Read the model definition and answer for the solid it produces. Units are mm, in the model's axes. A direction names the side the tool comes from. Round coordinates to 2 decimals unless told otherwise and drop trailing zeros. Order: outer loops, then holes, each group sorted by start corner. A loop starts at its lowest first (then second) coordinate and runs counter-clockwise, first axis right, second up. Notation, with made-up numbers: (12.5, 30) -> (61.5, 30) arc R19 cw to (61.5, 44) -> close; hole circle Ø9 at (7, 74). An arc over 180 degrees is marked (long way). Answer as a JSON object with one key per item and string values. Group by question number.
Item 1: Section C-C, the plane z = -15.75 is taken. Write down the section's boundary in (x, y), plus the area to 3 significant figures.
Item 2: For faces 1 (the flat face through (12.7, 72, -17)), 2 (the flat face through (-0.7, 5.1, -23)), 3 (the cylindrical face through (1.653, 121.812, -20.372)), determine the directions among +Z, -Z, +X, -X, +Y, -Y from which every point of the face is accessible in a straight line to the end or side of a thin tool.
Item 3: Section B-B, the plane z = -22.5 is taken. Write down the section's boundary in (x, y).
Item 4: The mould has two halves that part along Y. Classify faces 4 (the cylindrical face through (1.38, 103.02, -18.96)), 5 (the cylindrical face through (20.3, 14.9, -16.5)), 6 (the flat face through (0, 61, -12.7)): pulls with the +Y half, pulls with the -Y half, needs draft (parallel to the pull), parting line crosses it, or undercut.
Item 5: Consider probe 1 along X at (y, z) = (78, -17.5); probe 2 along Z at (x, y) = (5, 35); probe 3 along Y at (x, z) = (0, -17). Determine where each line is inside the solid, lowest interval first. Write a range as from..to.
Item 6: Section D-D, the plane y = 100.5 is taken. Write down the section's boundary in (x, z).
Item 7: Given P1, Ø1.5, axis at x = -39, z = -18, coming from the +Y side; P2, Ø12, axis at x = 12, y = 27, coming from the -Z side; P3, Ø14.5, axis at x = 0, y = 109.22, coming from the +Z side; P4, Ø4, axis at y = 72, z = -16, coming from the +X side, each flat-ended and moving along its own axis, determine where each tip first touches the part or whether it passes through.
from build123d import *

# Parameters (mm, degrees)
SKETCH1_R           = 6.35
BOSS_EXTRUDE1_DEPTH = 7.62
BOSS_EXTRUDE2_START = -5.08
SKETCH4_R           = 12.7
SKETCH4_R_2         = 6.35
BOSS_EXTRUDE2_DEPTH = 7.62
BOSS_EXTRUDE3_START = -5.08
SKETCH4_3_R         = 12.7
SKETCH4_3_R_2       = 6.35
BOSS_EXTRUDE3_DEPTH = 5.08
FILLET1_R           = 25.4
CHAMFER1_SIZE       = 4.92
CUT_EXTRUDE1_DEPTH  = 161.724006919


with BuildPart() as part:
    # Sketch1 → Boss-Extrude1 (new body)
    with BuildSketch(Plane(origin=(0, 0, 0), x_dir=(1, 0, 0), z_dir=(0, 1, 0))):
        with BuildLine():
            Line((-50.8, 25.4), (50.8, 25.4))
            Line((50.8, 25.4), (50.8, 0))
            ThreePointArc((50.8, 0), (43.360512242, -17.960512242), (25.4, -25.4))
            Line((25.4, -25.4), (-25.4, -25.4))
            ThreePointArc((-25.4, -25.4), (-43.360512242, -17.960512242), (-50.8, 0))
            Line((-50.8, 0), (-50.8, 25.4))
        make_face()
        with Locations(Location((-25.4, 0, 0), (0, 0, 90))):
            Circle(SKETCH1_R, mode=Mode.SUBTRACT)
        with Locations(Location((25.4, 0, 0), (0, 0, 90))):
            Circle(SKETCH1_R, mode=Mode.SUBTRACT)
    extrude(amount=BOSS_EXTRUDE1_DEPTH)

    # Sketch4 → Boss-Extrude2 (add)
    with BuildSketch(Plane(origin=(0, 0, -25.4), x_dir=(-1, 0, 0), z_dir=(0, 0, -1)).offset(BOSS_EXTRUDE2_START)):
        with BuildLine():
            Line((12.7, 7.62), (12.7, 109.22))
            ThreePointArc((12.7, 109.22), (0, 96.52), (-12.7, 109.22))
            Line((-12.7, 109.22), (-12.7, 7.62))
            Line((-12.7, 7.62), (12.7, 7.62))
        make_face()
        with Locations((0, 109.22)):
            Circle(SKETCH4_R)
        with Locations((0, 109.22)):
            Circle(SKETCH4_R_2, mode=Mode.SUBTRACT)
    extrude(amount=-BOSS_EXTRUDE2_DEPTH)

    # Sketch4_3 → Boss-Extrude3 (add)
    with BuildSketch(Plane(origin=(0, 0, -25.4), x_dir=(-1, 0, 0), z_dir=(0, 0, -1)).offset(BOSS_EXTRUDE3_START)):
        with Locations((0, 109.22)):
            Circle(SKETCH4_3_R)
        with Locations((0, 109.22)):
            Circle(SKETCH4_3_R_2, mode=Mode.SUBTRACT)
    extrude(amount=BOSS_EXTRUDE3_DEPTH)

    # Fillet1
    fillet1_edges = [part.edges().sort_by_distance(p)[0] for p in [
        (-12.7, 7.62, -16.51),
        (12.7, 7.62, -16.51),
    ]]
    fillet(fillet1_edges, radius=FILLET1_R)

    # Chamfer1
    chamfer1_edges = [part.edges().sort_by_distance(p)[0] for p in [
        (0, 7.62, -25.4),
    ]]
    chamfer(chamfer1_edges, length=CHAMFER1_SIZE)

    # Sketch8 → Cut-Extrude1 (cut, through all)
    with BuildSketch(Plane(origin=(50.8, 0, 0), x_dir=(0, 0, -1), z_dir=(1, 0, 0))):
        Polygon((12.717540877, 7.62), (20.337540877, 0), (-26.584534345, 0), (-26.584534345, 7.62), align=None)
    extrude(amount=-CUT_EXTRUDE1_DEPTH, mode=Mode.SUBTRACT)


solid = part.part
Values found:
{
 "1": {"outline": "(-50.8, 4.59) -> (50.8, 4.59) -> (50.8, 7.62) -> (38.1, 7.62) arc R25.4 cw to (12.7, 33.02) -> (12.7, 109.22) arc R12.7 ccw to (-12.7, 109.22) -> (-12.7, 33.02) arc R25.4 cw to (-38.1, 7.62) -> (-50.8, 7.62) -> close; hole circle Ø12.7 at (0, 109.22)", "area": "3,290 mm2"},
 "2": {"face 1": "+Z, -Z, +X, +Y", "face 2": "-Z, +X, -X", "face 3": "-Z"},
 "3": {"outline": "(-50.8, 0) -> (50.8, 0) -> (50.8, 5.6) -> (-50.8, 5.6) -> close; circle Ø25.4 at (0, 109.22); hole circle Ø12.7 at (0, 109.22)"},
 "4": {"face 4": "undercut", "face 5": "pulls with the +Y half", "face 6": "needs draft"},
 "5": {"probe 1": "-12.7..12.7", "probe 2": "-20.32..-12.7", "probe 3": "3.34..102.87, 115.57..121.92"},
 "6": {"outline": "(-12.7, -20.32) -> (-9.23, -20.32) -> (-9.23, -25.4) -> (9.23, -25.4) -> (9.23, -20.32) -> (12.7, -20.32) -> (12.7, -12.7) -> (-12.7, -12.7) -> close"},
 "7": {"P1": "y = 7.62", "P2": "z = -20.32", "P3": "z = -12.7", "P4": "x = 12.7"}
}
